Build history of the part. All positions in model axes, mm. Face numbers are marked on the shaded views. A direction names the side the tool comes from. Give positions to 0.01 mm unless a question says otherwise; leave off trailing zeros. Order: outer loops, then holes, each group sorted by start corner. A loop starts at its lowest first (then second) coordinate and runs counter-clockwise, first axis right, second up. Notation, with made-up numbers: (74, -4.75) -> (116, -4.75) arc R16 cw to (116, 24.25) -> close; hole circle Ø9 at (-3.5, 62). An arc over 180 degrees is marked (long way). Write item = value, one per line. Start each with the question number.
from build123d import *

# Parameters (mm, degrees)
SKETCH1_W           = 19.05
SKETCH1_H           = 44.45
BOSS_EXTRUDE1_DEPTH = 5.08
SKETCH2_W           = 25.4
SKETCH2_H           = 50.8
BOSS_EXTRUDE2_DEPTH = 3.175
FILLET1_R           = 3.175


with BuildPart() as part:
    # Sketch1 → Boss-Extrude1 (new body)
    with BuildSketch(Plane(origin=(0, 0, 0), x_dir=(1, 0, 0), z_dir=(0, 1, 0))):
        Rectangle(SKETCH1_W, SKETCH1_H)
    extrude(amount=BOSS_EXTRUDE1_DEPTH)

    # Sketch2 → Boss-Extrude2 (add)
    with BuildSketch(Plane(origin=(0, 5.08, 0), x_dir=(1, 0, 0), z_dir=(0, 1, 0))):
        Rectangle(SKETCH2_W, SKETCH2_H)
    extrude(amount=BOSS_EXTRUDE2_DEPTH)

    # Fillet1
    fillet1_edges = [part.edges().sort_by_distance(p)[0] for p in [
        (0, 8.255, -25.4),
        (-12.7, 8.255, 0),
        (0, 8.255, 25.4),
        (12.7, 8.255, 0),
    ]]
    fillet(fillet1_edges, radius=FILLET1_R - 0.0001)  # a hair under: the kernel refuses the full size


solid = part.part
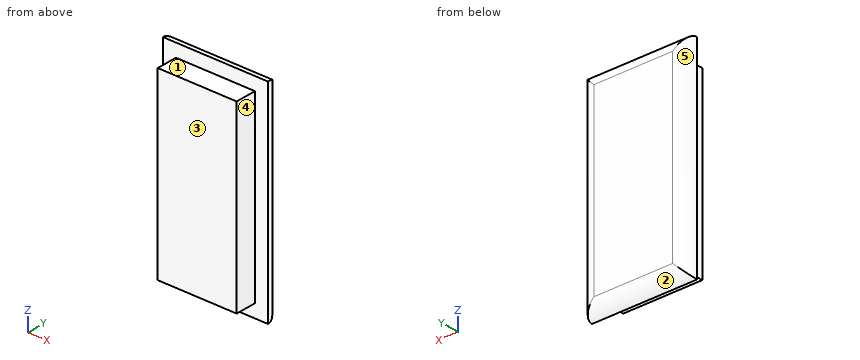
(1) Mould opens along Z. For the marked faces 1, 2 and 3 say: released by +Z, released by -Z, zero draft, split by the parting line, or undercut.
(2) Wall check: line 1 (X direction, y = 4, z = -14) (3 decimals); line 2 (Z direction, x = 5.75, y = 3.5) (3 decimals); line 3 (Z direction, x = 10.5, y = 5.25). Give the ranges that are in metal, low to high. Write a range as [from, to].
(3) 3-axis set-ups, long thin cutter, end or side, ignore diameter. For the marked faces 4 and 5: which of +Z, -Z, +X, -X, +Y, -Y reach the whole face in a straight line?
(4) Flat gauge pins, fed straight in: P1, Ø2, axis at y = 3.5, z = 2, coming from the -X side (3 decimals); P2, Ø1.5, axis at x = 0, y = 3.5, coming from the +Z side (3 decimals); P3, Ø2.5, axis at x = 1, y = 3.5, coming from the -Z side (3 decimals). Where does each tip first touch, or does it go through?
(5) Cut at C-C, the plane y = 1. Give the cut face in (x, z) (3 decimals), plus the area to 3 significant figures.
Results:
q1.face_1 = released by +Z
q1.face_2 = released by -Z
q1.face_3 = zero draft
q2.line_1 = [-9.525, 9.525]
q2.line_2 = [-22.225, 22.225]
q2.line_3 = [-25.4, 25.4]
q3.face_4 = +Z, -Z, +X, -Y
q3.face_5 = +Z, -Z, -X, +Y
q4.P1 = -9.525
q4.P2 = 22.225
q4.P3 = -22.225
q5.outline = (-9.525, -22.225) -> (9.525, -22.225) -> (9.525, 22.225) -> (-9.525, 22.225) -> close
q5.area = 847 mm2
